Check sheet for the modelled part. Datum: model origin and axes. Units: mm. Face numbers are marked on the shaded views. A direction names the side the tool comes from. Give positions to 0.01 mm unless a question says otherwise; leave off trailing zeros. Order: outer loops, then holes, each group sorted by start corner. A loop starts at its lowest first (then second) coordinate and runs counter-clockwise, first axis right, second up. Notation, with made-up numbers: (34.25, 62) - (73.25, 62) arc R19 ccw to (73.25, 93) - close; hole circle Ø6 at (48, -34). An arc over 180 degrees is marked (long way). Answer in a Markdown table with one row per item.
Autodesk Inventor part; units mm, degrees
ref_plane "YZ Plane" through (0, 0, 0) normal (1, 0, 0) x (0, 1, 0)
ref_plane "XZ Plane" through (0, 0, 0) normal (0, 1, 0) x (-1, 0, 0)
ref_plane "XY Plane" through (0, 0, 0) normal (0, 0, 1) x (1, 0, 0)
sketch "Sketch1" plane through (0, 0, 0) normal (0, 0, 1) x (1, 0, 0)
  circle A0 centre (0, 0) radius 14
  circle A1 centre (0, 0) radius 17
  dimension "d0" = 28
  dimension "d2" = 34
extrude "Extrusion1" add sketch "Sketch1" along normal blind 6.8
sketch "Sketch2" plane through (0, 0, 6.8) normal (0, 0, 1) x (1, 0, 0)
  circle A0 centre (0, 0) radius 17
extrude "Extrusion2" add sketch "Sketch2" along normal blind 4
sketch "Sketch3" plane through (0, 0, 10.8) normal (0, 0, 1) x (1, 0, 0)
  circle A0 centre (0, 0) radius 17
  circle A1 centre (0, 0) radius 9
  dimension "d7" = 18
extrude "Extrusion3" cut sketch "Sketch3" against normal blind 4 contours A1
properties part number "Bearing cap"
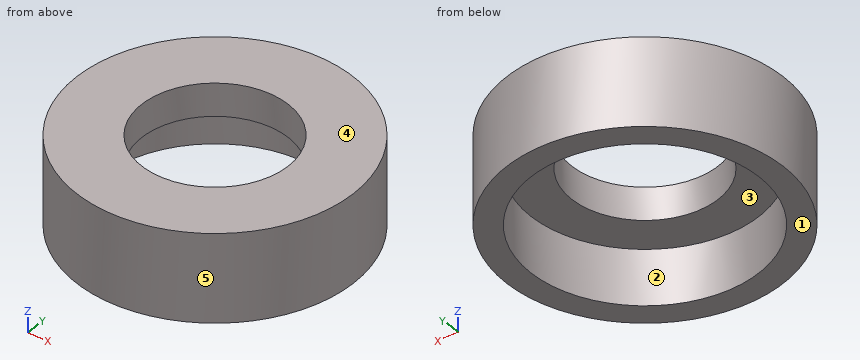
(1) Cross-section at C-C, the plane z = 5.5. Record the cut outline in (x, y).
Geometry says:
| item | result |
|---|---|
| outline | circle Ø34 at (0, 0); hole circle Ø28 at (0, 0) |
(2) Access from +Z, -Z, +X, -X, +Y, -Y to the whole of each face (thin tool, end or side, straight path). Record for the marked faces 1 and 2.
Geometry says:
| item | result |
|---|---|
| face 1 | -Z, +X, -X, +Y, -Y |
| face 2 | -Z |
(3) Cross-section at A-A, the plane y = 0. Record the cut outline in (x, z), then the cut area to 3 significant figures.
Geometry says:
| item | result |
|---|---|
| outline | (-17, 0) - (-14, 0) - (-14, 6.8) - (-9, 6.8) - (-9, 10.8) - (-17, 10.8) - close; (9, 6.8) - (14, 6.8) - (14, 0) - (17, 0) - (17, 10.8) - (9, 10.8) - close |
| area | 105 mm² |
(4) Thickness scan on L1, parallel to Y at x = 0, z = 7.25; L2, parallel to Y at x = 0, z = 4.25; L3, parallel to Z at x = -9, y = -5. Record the ranges inside material, lowest first.
Geometry says:
| item | result |
|---|---|
| L1 | -17 to -9, 9 to 17 |
| L2 | -17 to -14, 14 to 17 |
| L3 | 6.8 to 10.8 |
(5) Gauge pin test, flat ends, axial feed: P1, Ø6, axis at y = -7.5, z = 3, coming from the +X side; P2, Ø5, axis at x = 11.5, z = 1, coming from the +Y side; P3, Ø2, axis at y = 7.5, z = 8.5, coming from the -X side. Record the tip position at first contact, or that the pin passes through.
Geometry says:
| item | result |
|---|---|
| P1 | x = 16.39 |
| P2 | y = 14.42 |
| P3 | x = -15.71 |
(6) Cross-section at D-D, the plane x = 13.5. Record the cut outline in (y, z).
Geometry says:
| item | result |
|---|---|
| outline | (-10.33, 0) - (-3.71, 0) - (-3.71, 6.8) - (3.71, 6.8) - (3.71, 0) - (10.33, 0) - (10.33, 10.8) - (-10.33, 10.8) - close |
(7) Mould release check, pull along Y, two halves, no side actions. Record for the marked faces 3, 4 and 5: pulls with the +Y half, pulls with the -Y half, needs draft (parallel to the pull), parting line crosses it, or undercut.
Geometry says:
| item | result |
|---|---|
| face 3 | undercut |
| face 4 | needs draft |
| face 5 | parting line crosses it |
